from build123d import *

# Parameters (mm, degrees)
SKETCH1_W           = 70
SKETCH1_H           = 70
SKETCH1_W_2         = 34.5
SKETCH1_H_2         = 36
BOSS_EXTRUDE1_DEPTH = 2
SKETCH2_W           = 2
SKETCH2_H           = 20
SKETCH2_W_2         = 20
SKETCH2_H_2         = 2
CUT_EXTRUDE1_DEPTH  = 2


with BuildPart() as part:
    # Sketch1 → Boss-Extrude1 (new body)
    with BuildSketch(Plane.XY):
        Rectangle(SKETCH1_W, SKETCH1_H)
        Rectangle(SKETCH1_W_2, SKETCH1_H_2, mode=Mode.SUBTRACT)
    extrude(amount=-BOSS_EXTRUDE1_DEPTH)

    # Sketch2 → Cut-Extrude1 (cut)
    with BuildSketch(Plane.XY):
        with Locations((-34, 15)):
            Rectangle(SKETCH2_W, SKETCH2_H)
        with Locations((-34, -15)):
            Rectangle(SKETCH2_W, SKETCH2_H)
        with Locations((-15, -34)):
            Rectangle(SKETCH2_W_2, SKETCH2_H_2)
        with Locations((15, -34)):
            Rectangle(SKETCH2_W_2, SKETCH2_H_2)
        with Locations((34, -15)):
            Rectangle(SKETCH2_W, SKETCH2_H)
        with Locations((34, 15)):
            Rectangle(SKETCH2_W, SKETCH2_H)
        with Locations((15, 34)):
            Rectangle(SKETCH2_W_2, SKETCH2_H_2)
        with Locations((-15, 34)):
            Rectangle(SKETCH2_W_2, SKETCH2_H_2)
    extrude(amount=-CUT_EXTRUDE1_DEPTH, mode=Mode.SUBTRACT)


solid = part.part
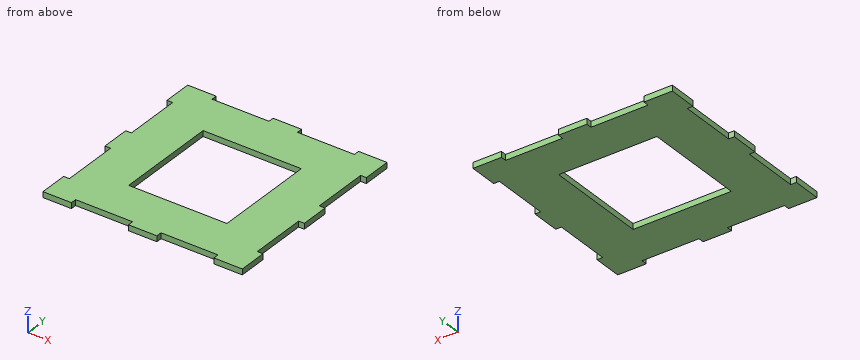
Could you check a few things on this model? Use its own coordinates, in mm. Give positions to 0.01 mm unless a question says otherwise; leave off trailing zeros. Order: outer loops, then holes, each group sorted by start corner. A loop starts at its lowest first (then second) coordinate and runs counter-clockwise, first axis right, second up.
Item 1: If we section it at C-C, the plane y = -22.5: Write out the boundary of the cut face in (x, z).
Item 2: If we section it at A-A, the plane x = 3.5: Write out the boundary of the cut face in (y, z), plus the area to 3 significant figures.
Item 3: I'm going to push flat-ended pins straight in: pin 1 (0.6 mm diameter, centred on x = 6, z = -0.5, fed in from +Y); pin 2 (1 mm diameter, centred on y = 18.5, z = -1, fed in from +X); pin 3 (1 mm diameter, centred on y = -14, z = -1.5, fed in from -X). Where does each tip first touch, or does it pass through?
Item 4: If we section it at B-B, the plane y = -3: Write out the boundary of the cut face in (x, z), plus the area to 3 significant figures.
Item 5: I need wall thicknesses on line 1 (X direction, y = -16.5, z = -0.25); line 2 (Y direction, x = -1.5, z = -1.85); line 3 (X direction, y = 1, z = -0.65). Which ranges of each line are inside material? Lowest first, please.
Values:
1. outline: (-33, -2) - (33, -2) - (33, 0) - (-33, 0) - close
2. outline: (-35, -2) - (-18, -2) - (-18, 0) - (-35, 0) - close; (18, -2) - (35, -2) - (35, 0) - (18, 0) - close
2. area: 68.0 mm2
3. pin 1: stops at y = 33
3. pin 2: stops at x = 33
3. pin 3: stops at x = -33
4. outline: (-35, -2) - (-17.25, -2) - (-17.25, 0) - (-35, 0) - close; (17.25, -2) - (35, -2) - (35, 0) - (17.25, 0) - close
4. area: 71.0 mm2
5. line 1: x = -33 to -17.25, 17.25 to 33
5. line 2: y = -35 to -18, 18 to 35
5. line 3: x = -35 to -17.25, 17.25 to 35
